```python
from build123d import *

# Parameters (mm, degrees)
F0_W     = 79.648294
F0_H     = 25.750952
F1_DEPTH = 50
F2_W     = 57.916386
F2_H     = 24.148573
F3_DEPTH = 25
F4_R     = 0.5
F5_DEPTH = 10


with BuildPart() as f1:
    # F0 (on Top) → F1 (new body)
    with BuildSketch(Plane.XY):
        Rectangle(F0_W, F0_H)
    extrude(amount=F1_DEPTH)

    # F2 (on face) → F3 (cut)
    with BuildSketch(Plane.XY.offset(50)):
        with Locations((-9.955351, 0.343398)):
            Rectangle(F2_W, F2_H)
    extrude(amount=-F3_DEPTH, mode=Mode.SUBTRACT)

    # F4 (on face) → F5 (join)
    with BuildSketch(Plane.XY.offset(50)):
        with Locations((29.824147, 0)):
            Circle(F4_R)
    extrude(amount=F5_DEPTH)


solid = f1.part
```
Source: CAD feature listing. Evaluate the final solid. Frame: model axes, mm. A direction names the side the tool comes from. Give positions to 0.01 mm unless a question says otherwise; leave off trailing zeros. Order: outer loops, then holes, each group sorted by start corner. A loop starts at its lowest first (then second) coordinate and runs counter-clockwise, first axis right, second up.
(1) Section query C-C (x = -0.5). Return the cut outline in (y, z), plus the area to 3 significant figures.
(2) Pull-direction query (Y, two-part tool) for faces 1 (the face through (-1, -12.875, 25)), 2 (the face through (-39.824, 0, 25)), 3 (the face through (-10, -11.731, 38)); classes: +Y half, -Y half, draft (parallel to the pull), parting line (faces both ways), or undercut.
(3) Material intervals for line 1 along X through (y, z) = (7, 35); line 2 along Y through (x, z) = (-29, 43.5); line 3 along Z through (x, y) = (-15, -3.75), sorted ascending.
(4) Section query B-B (y = 3.25). Return the cut outline in (x, z), plus the area to 3 significant figures.
(5) Access query for faces 4 (the face through (19.003, 0, 38)), 5 (the face through (-1, 12.875, 25)). Directions: +Z, -Z, +X, -X, +Y, -Y. A direction counts if a zero-diameter tool reaches every point of the face in a straight line with its end or side. Return the directions, or none.
(6) Section query A-A (z = 34). Return the cut outline in (x, y), plus the area to 3 significant figures.
(7) Contact query for flat-ended pins moving along their axis: P1, Ø7.5, axis at x = -12.5, y = 0.5, coming from the +Z side; P2, Ø12, axis at x = 26, y = 7.5, coming from the +Z side. Output: stop coordinate, or through.
Outcome:
1. outline: (-12.88, 0) - (12.88, 0) - (12.88, 50) - (12.42, 50) - (12.42, 25) - (-11.73, 25) - (-11.73, 50) - (-12.88, 50) - close
1. area: 684 mm2
2. face 1: -Y half
2. face 2: draft
2. face 3: undercut
3. line 1: x = -39.82 to -38.91, 19 to 39.82
3. line 2: y = -12.88 to -11.73, 12.42 to 12.88
3. line 3: z = 0 to 25
4. outline: (-39.82, 0) - (39.82, 0) - (39.82, 50) - (19, 50) - (19, 25) - (-38.91, 25) - (-38.91, 50) - (-39.82, 50) - close
4. area: 2,530 mm2
5. face 4: +Z
5. face 5: +Z, -Z, +X, -X, +Y
6. outline: (-39.82, -12.88) - (39.82, -12.88) - (39.82, 12.88) - (-39.82, 12.88) - close; hole (-38.91, -11.73) - (19, -11.73) - (19, 12.42) - (-38.91, 12.42) - close
6. area: 652 mm2
7. P1: stops at z = 25
7. P2: stops at z = 50
